from build123d import *

# Parameters (mm, degrees)
BOSS_EXTRUDE1_DEPTH = 500
FILLET1_R           = 12


with BuildPart() as part:
    # Sketch1 → Boss-Extrude1 (new body)
    with BuildSketch(Plane.XY):
        Polygon((-40, 16.25), (-40, -18.75), (40, -18.75), (40, 16.25), (35, 16.25), (35, -10.594931419), (27.223611076, -10.594931419), (0, 16.628679656), (-27.223611076, -10.594931419), (-35, -10.594931419), (-35, 16.25), align=None)
    extrude(amount=BOSS_EXTRUDE1_DEPTH)

    # Fillet1
    fillet1_edges = [part.edges().sort_by_distance(p)[0] for p in [
        (0, 16.628679656, 250),
    ]]
    fillet(fillet1_edges, radius=FILLET1_R)


solid = part.part
The model under review builds one solid part; all positions refer to its coordinate system, in mm. A direction names the side the tool comes from. Give positions to 0.01 mm unless a question says otherwise; leave off trailing zeros. Order: outer loops, then holes, each group sorted by start corner. A loop starts at its lowest first (then second) coordinate and runs counter-clockwise, first axis right, second up. Notation, with made-up numbers: (60.5, 7) -> (80.5, 7) arc R25 ccw to (80.5, 44) -> close; hole circle Ø1 at (-31, 34). An arc over 180 degrees is marked (long way). Write item = value, one per line. Start each with the question number.
(1) Tool access review of faces 1 (the flat face through (-9, -5, 0)), 2 (the flat face through (35, 3, 246)): name each direction out of +Z, -Z, +X, -X, +Y, -Y from which nothing blocks a thin tool from reaching the whole face with its end or side.
(2) Take a section at D-D (x = -2.5). Write out the cut boundary in (y, z), plus the area to 3 significant figures.
(3) For L1, parallel to X at y = -8.5, z = 320.5; L2, parallel to X at y = -10.5, z = 186.5; L3, parallel to Y at x = -28.5, z = 476, list the stretches that pass through material, from the lowest coordinate up. Write a range as from..to.
(4) Take a section at B-B (z = 375). Write out the cut boundary in (x, y).
(5) Take a section at A-A (y = 1.5). Write out the cut boundary in (x, z), plus the area to 3 significant figures.
(6) For pin 1 Ø1 at (x, z) = (31.5, 177) entering from +Y; pin 2 Ø4 at (x, z) = (11, 230.5) entering from +Y; pin 3 Ø8.5 at (x, z) = (30.5, 287.5) entering from +Y, all flat-tipped, find the tip position at first contact; note any pin that passes through.
(7) Take a section at C-C (x = 18.5). Write out the cut boundary in (y, z).
(8) Draft analysis for pull direction X (two halves, no side actions). For faces 3 (the flat face through (-40, -1, 246)), 4 (the flat face through (-9, -5, 500)), 5 (the flat face through (-35, 3, 246)), state which applies: +X half, -X half, draft (parallel to the pull), parting line (faces both ways), or undercut.
Returned:
q1.face_1 = -Z, +X, -X, +Y, -Y
q1.face_2 = +Z, -Z, +Y
q2.outline = (-18.75, 0) -> (11.39, 0) -> (11.39, 500) -> (-18.75, 500) -> close
q2.area = 15,100 mm²
q3.L1 = -40..-35, -25.13..25.13, 35..40
q3.L2 = -40..-35, -27.13..27.13, 35..40
q3.L3 = -18.75..-10.59
q4.outline = (-40, -18.75) -> (40, -18.75) -> (40, 16.25) -> (35, 16.25) -> (35, -10.59) -> (27.22, -10.59) -> (8.49, 8.14) arc R12 ccw to (-8.49, 8.14) -> (-27.22, -10.59) -> (-35, -10.59) -> (-35, 16.25) -> (-40, 16.25) -> close
q5.outline = (-40, 0) -> (-35, 0) -> (-35, 500) -> (-40, 500) -> close; (-15.13, 0) -> (15.13, 0) -> (15.13, 500) -> (-15.13, 500) -> close; (35, 0) -> (40, 0) -> (40, 500) -> (35, 500) -> close
q5.area = 20,100 mm²
q6.pin_1 = -10.59
q6.pin_2 = 7.63
q6.pin_3 = -9.62
q7.outline = (-18.75, 0) -> (-1.87, 0) -> (-1.87, 500) -> (-18.75, 500) -> close
q8.face_3 = -X half
q8.face_4 = draft
q8.face_5 = undercut
